Drawing for the job (mm, zero at the part's lowest x, y, z). A direction names the side the tool comes from. Give positions to 0.01 mm unless a question says otherwise; leave off trailing zeros. Loops run counter-clockwise (first coordinate to the right, second up) from the corner with the lowest first, then second, coordinate; pieces in that order, holes last.
1) Flat gauge pins, fed straight in: P1, Ø5, axis at x = 13, y = 9.5, coming from the -Z side; P2, Ø4, axis at x = 39.5, y = 7.5, coming from the +Z side; P3, Ø2, axis at x = 38, y = 5.5, coming from the -Z side; P4, Ø4, axis at x = 6.5, y = 3, coming from the -Z side. Where does each tip first touch, or does it go through?
2) Two-plate mould, pull along X, no slides. Class the marked faces 1, 2 and 3: +X half, -X half, draft (parallel to the pull), parting line (faces both ways), or undercut.
3) Wall check: line 1 (X direction, y = 7.5, z = 20.75); line 2 (Y direction, x = 39.5, z = 36); line 3 (X direction, y = 10.75, z = 7.5). Give the ranges that are in metal, low to high.
4) 3-axis set-ups, long thin cutter, end or side, ignore diameter. For the marked faces 4 and 5: which of +Z, -Z, +X, -X, +Y, -Y reach the whole face in a straight line?
5) Band-saw the part on C-C on y = 7.5. List the corners of the cut face in (x, z).
6) Band-saw the part on B-B on x = 39.5. List the corners of the cut face in (y, z), then the cut area to 3 significant figures.
7) Band-saw the part on D-D on z = 14. List the corners of the cut face in (x, y), then the cut area to 3 significant figures.
8) Band-saw the part on A-A on z = 9.5. List the corners of the cut face in (x, y).
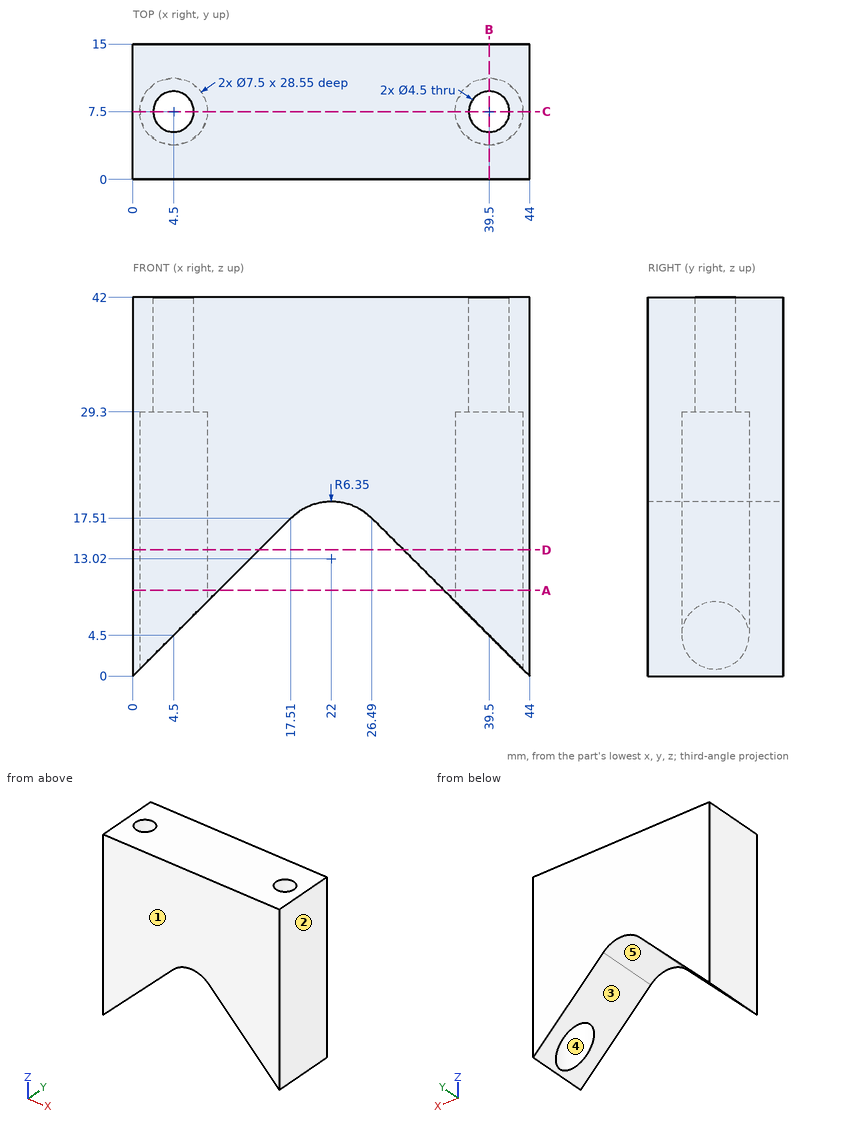
Findings below:
1. P1: stops at z = 10.5
1. P2: passes through
1. P3: stops at z = 29.3
1. P4: stops at z = 4.5
2. face 1: draft
2. face 2: +X half
2. face 3: undercut
3. line 1: x = 0 to 0.75, 8.25 to 35.75, 43.25 to 44
3. line 2: y = 0 to 5.25, 9.75 to 15
3. line 3: x = 0 to 2.63, 6.37 to 7.5, 36.5 to 37.63, 41.37 to 44
4. face 4: -Z
4. face 5: -Z, +Y, -Y
5. outline: (0, 0) - (0.75, 0.75) - (0.75, 29.3) - (2.25, 29.3) - (2.25, 42) - (0, 42) - close; (6.75, 29.3) - (8.25, 29.3) - (8.25, 8.25) - (17.51, 17.51) arc R6.35 cw to (26.49, 17.51) - (35.75, 8.25) - (35.75, 29.3) - (37.25, 29.3) - (37.25, 42) - (6.75, 42) - close; (41.75, 29.3) - (43.25, 29.3) - (43.25, 0.75) - (44, 0) - (44, 42) - (41.75, 42) - close
6. outline: (0, 4.5) - (3.75, 4.5) - (3.75, 29.3) - (5.25, 29.3) - (5.25, 42) - (0, 42) - close; (9.75, 29.3) - (11.25, 29.3) - (11.25, 4.5) - (15, 4.5) - (15, 42) - (9.75, 42) - close
6. area: 319 mm2
7. outline: (0, 0) - (14, 0) - (14, 15) - (0, 15) - close; (30, 0) - (44, 0) - (44, 15) - (30, 15) - close; hole circle Ø7.5 at (4.5, 7.5); hole circle Ø7.5 at (39.5, 7.5)
7. area: 332 mm2
8. outline: (0, 0) - (9.5, 0) - (9.5, 15) - (0, 15) - close; (34.5, 0) - (44, 0) - (44, 15) - (34.5, 15) - close; hole circle Ø7.5 at (4.5, 7.5); hole circle Ø7.5 at (39.5, 7.5)
